Can you work these out from the model? Positions are in its coordinate system, mm. A direction names the side the tool comes from. Round coordinates to 2 decimals unless told otherwise and drop trailing zeros. Write each loop counter-clockwise with the first axis right and the second up, starting at its lowest first coordinate (ties: lowest second). Pieces come first, ordered by that corner, then holes. Notation, with made-up numbers: (-25.5, -11.5) - (25.5, -11.5) arc R21 ccw to (25.5, 16.5) - close; hole circle Ø2 at (43, -6). An arc over 180 degrees is marked (long way). One line per item, written item: value. Start each with the question number.
(1) I want a section at C-C on y = -31. List the corners of the cut face in (x, z) for me.
(2) I'm going to push flat-ended pins straight in: pin 1 Ø6 at (y, z) = (-14, 17) entering from -X; pin 2 Ø8 at (x, y) = (64, -40.5) entering from +Z; pin 3 Ø6.5 at (x, z) = (69.5, 9.5) entering from -Y. Where does each tip first touch, or does it pass through?
(3) If I drill on L1, parallel to Y at x = 38.1, z = 18; L2, parallel to Z at x = 6.35, y = -2.75; L3, parallel to X at y = -6, z = 15, over which ranges is the centre line in solid material (lowest first)? Write a range as from..to.
(4) I want a section at A-A on z = 12.7. List the corners of the cut face in (x, y) for me.
(5) Thinking about a two-plate mould opening in Z: for faces 4 (the face through (5.93, -3.22, 15.91)), 5 (the face through (66.615, -3.219, 12.842)), 6 (the face through (38, -25, 25.4)), 7 (the face through (12.703, -28, 13)), which applies, +Z half, -Z half, draft (parallel to the pull), parting line (faces both ways), or undercut?
(6) I want a section at D-D on z = 8. List the corners of the cut face in (x, y) for me, plus the area to 3 significant figures.
(7) On a 3-axis mill with a long thin cutter (end or side, diameter ignored), from which of +Z, -Z, +X, -X, +Y, -Y can I reach the whole of each face in a straight line? I mean faces 1 (the face through (76.2, -3, 13)), 2 (the face through (63.5, -29, 13)), 3 (the face through (3, -6.35, 10)). Say none if no direction works.
(8) I want a section at B-B on x = 69.85. List the corners of the cut face in (y, z) for me, plus the area to 3 significant figures.
from build123d import *

# Parameters (mm, degrees)
F1_DEPTH = 25.4
F4_R     = 3.2385
F5_DEPTH = 25.4
F3_R     = 3.2385
F6_DEPTH = 25.4
F8_D     = 7.9375


with BuildPart() as f1:
    # F0 (on Top) → F1 (new body)
    with BuildSketch(Plane.XY):
        Polygon((76.2, 0), (0, 0), (0, -6.35), (12.7030108124, -6.35), (12.7030108124, -50.8), (63.5, -50.8), (63.5, -6.35), (76.2, -6.35), align=None)
    extrude(amount=F1_DEPTH)

    # F4 (on face) → F5 (cut)
    with BuildSketch(Plane.XZ.offset(6.35)):
        with Locations((6.35, 12.7)):
            Circle(F4_R)
    extrude(amount=-F5_DEPTH, mode=Mode.SUBTRACT)

    # F3 (on face) → F6 (cut)
    with BuildSketch(Plane.XZ.offset(6.35)):
        with Locations((69.85, 12.7)):
            Circle(F3_R)
    extrude(amount=-F6_DEPTH, mode=Mode.SUBTRACT)

    # F8 (through all)
    with Locations(Plane.XY.offset(25.4)):
        with Locations((38.1, -33.3375)):
            Hole(F8_D / 2)


solid = f1.part
Established:
1. outline: (12.7, 0) - (34.89, 0) - (34.89, 25.4) - (12.7, 25.4) - close; (41.31, 0) - (63.5, 0) - (63.5, 25.4) - (41.31, 25.4) - close
2. pin 1: x = 12.7
2. pin 2: z = 25.4
2. pin 3: y = -6.35
3. L1: -50.8..-37.31, -29.37..0
3. L2: 0..9.46, 15.94..25.4
3. L3: 0..4.07, 8.63..67.57, 72.13..76.2
4. outline: (0, -6.35) - (3.11, -6.35) - (3.11, 0) - (0, 0) - close; (9.59, -6.35) - (12.7, -6.35) - (12.7, -50.8) - (63.5, -50.8) - (63.5, -6.35) - (66.61, -6.35) - (66.61, 0) - (9.59, 0) - close; (73.09, -6.35) - (76.2, -6.35) - (76.2, 0) - (73.09, 0) - close; hole circle Ø7.94 at (38.1, -33.34)
5. face 4: undercut
5. face 5: undercut
5. face 6: +Z half
5. face 7: draft
6. outline: (0, -6.35) - (12.7, -6.35) - (12.7, -50.8) - (63.5, -50.8) - (63.5, -6.35) - (76.2, -6.35) - (76.2, 0) - (0, 0) - close; hole circle Ø7.94 at (38.1, -33.34)
6. area: 2,690 mm2
7. face 1: +Z, -Z, +X, +Y, -Y
7. face 2: +Z, -Z, +X, -Y
7. face 3: +Z, -Z, -X, -Y
8. outline: (-6.35, 0) - (0, 0) - (0, 9.46) - (-6.35, 9.46) - close; (-6.35, 15.94) - (0, 15.94) - (0, 25.4) - (-6.35, 25.4) - close
8. area: 120 mm2
